Here's how the part is built. I have some questions about the finished solid (model axes, mm). Coordinates: 2 decimals unless noted, no trailing zeros. Loops run counter-clockwise (first coordinate to the right, second up) from the corner with the lowest first, then second, coordinate; pieces in that order, holes last.
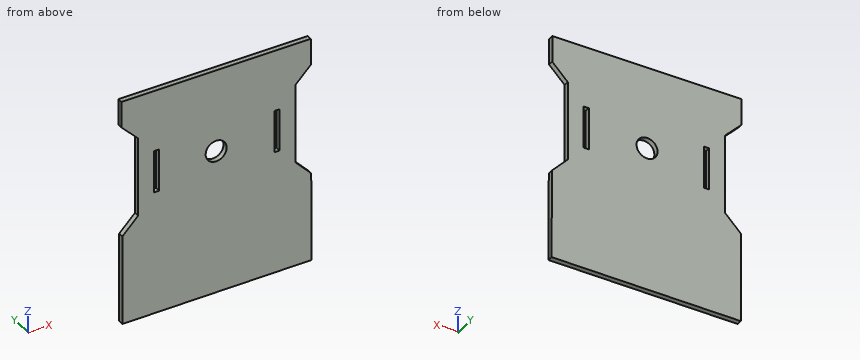
```python
from build123d import *

# Parameters (mm, degrees)
BOSS_EXTRUDE1_DEPTH = 5
CUT_EXTRUDE2_DEPTH  = 5
SKETCH5_W           = 5
SKETCH5_H           = 40
CUT_EXTRUDE3_DEPTH  = 10
SKETCH6_R           = 10
CUT_EXTRUDE4_DEPTH  = 10


with BuildPart() as part:
    # Sketch2 → Boss-Extrude1 (new body)
    with BuildSketch(Plane(origin=(0, 0, 0), x_dir=(1, 0, 0), z_dir=(0, 1, 0))):
        Polygon((-124.760229314, 128.809560066), (55.239770686, 127.913370731), (54.741887722, 27.913370731), (39.741887722, 27.913370731), (39.741887722, -47.086629269), (54.542734536, -61.887476084), (54.418263795, -86.887476084), (-125.581736205, -86.887476084), (-125.457265464, -61.887476084), (-109.760229314, -46.190439934), (-109.760229314, 28.809560066), (-124.760229314, 28.809560066), align=None)
    extrude(amount=BOSS_EXTRUDE1_DEPTH)

    # Sketch4 → Cut-Extrude2 (cut)
    with BuildSketch(Plane(origin=(0, 5, 0), x_dir=(1, 0, 0), z_dir=(0, 1, 0))):
        Polygon((-109.760229314, 28.809560066), (-124.760229314, 43.809560066), (-124.760229314, 28.809560066), align=None)
        Polygon((39.741887722, 27.913370731), (54.820327412, 43.668014969), (54.741887722, 27.913370731), align=None)
    extrude(amount=-CUT_EXTRUDE2_DEPTH, mode=Mode.SUBTRACT)

    # Sketch5 → Cut-Extrude3 (cut)
    with BuildSketch(Plane(origin=(0, 5, 0), x_dir=(1, 0, 0), z_dir=(0, 1, 0))):
        with Locations((-92.260229314, -8.690439934)):
            Rectangle(SKETCH5_W, SKETCH5_H)
        with Locations((22.241887722, -8.690439934)):
            Rectangle(SKETCH5_W, SKETCH5_H)
    extrude(amount=-CUT_EXTRUDE3_DEPTH, mode=Mode.SUBTRACT)

    # Sketch6 → Cut-Extrude4 (cut)
    with BuildSketch(Plane(origin=(0, 5, 0), x_dir=(1, 0, 0), z_dir=(0, 1, 0))):
        with Locations(Location((-35.581736205, -8.690439934, 0), (0, 0, 270))):
            Circle(SKETCH6_R)
    extrude(amount=-CUT_EXTRUDE4_DEPTH, mode=Mode.SUBTRACT)


solid = part.part
```
1. I want a section at A-A (z = -5). Please give me the cut outline in (x, y).
2. For pin 1 (2 mm diameter, centred on y = 3, z = 11, fed in from -X); pin 2 (1.5 mm diameter, centred on x = 22, y = 3, fed in from -Z); pin 3 (12 mm diameter, centred on x = -29, z = -26, fed in from -Y); pin 4 (2.5 mm diameter, centred on y = 3.5, z = -107, fed in from -X), each with a flat end and sliding along its axis, tell me the tip position at first contact or that it passes through.
3. I need wall thicknesses on line 1 along X through (y, z) = (2.5, -118); line 2 along X through (y, z) = (3.05, -67); line 3 along Z through (x, y) = (-11.5, 3.25). Which ranges of each line are inside material? Lowest first, please.
4. I want a section at C-C (x = -38). Please give me the cut outline in (y, z).
5. I want a section at B-B (y = 4.25). Please give me the cut outline in (x, z), then the cut area to 3 significant figures.
Response values:
1. outline: (-109.76, 0) - (-94.76, 0) - (-94.76, 5) - (-109.76, 5) - close; (-89.76, 0) - (19.74, 0) - (19.74, 5) - (-89.76, 5) - close; (24.74, 0) - (39.74, 0) - (39.74, 5) - (24.74, 5) - close
2. pin 1: stops at x = -109.76
2. pin 2: stops at z = -128.08
2. pin 3: stops at y = 0
2. pin 4: stops at x = -124.76
3. line 1: x = -124.76 to 55.19
3. line 2: x = -124.76 to 54.94
3. line 3: z = -128.25 to 86.89
4. outline: (0, -128.38) - (5, -128.38) - (5, -1.01) - (0, -1.01) - close; (0, 18.39) - (5, 18.39) - (5, 86.89) - (0, 86.89) - close
5. outline: (-125.58, 86.89) - (-125.46, 61.89) - (-109.76, 46.19) - (-109.76, -28.81) - (-124.76, -43.81) - (-124.76, -128.81) - (55.24, -127.91) - (54.82, -43.67) - (39.74, -27.91) - (39.74, 47.09) - (54.54, 61.89) - (54.42, 86.89) - close; hole (-94.76, -11.31) - (-89.76, -11.31) - (-89.76, 28.69) - (-94.76, 28.69) - close; hole circle Ø20 at (-35.58, 8.69); hole (19.74, -11.31) - (24.74, -11.31) - (24.74, 28.69) - (19.74, 28.69) - close
5. area: 35,300 mm2
